from build123d import *

# Parameters (mm, degrees)
F2_R     = 5
F4_DEPTH = 1


with BuildPart() as f1:
    # F0 (on Front) → F1 (revolve)
    with BuildSketch(Plane.XZ):
        with BuildLine():
            Line((-25, 14.134617), (-25, 0))
            Line((-25, 0), (0, 0))
            Line((0, 0), (0, 35))
            ThreePointArc((0, 35), (-5.59017, 33.68034), (-10, 30))
            Line((-10, 30), (-17.5, 30))
            Line((-17.5, 30), (-17.5, 14.134617))
            Line((-17.5, 14.134617), (-25, 14.134617))
        make_face()
    revolve(axis=Axis((0, 0, 17.5), (0, 0, 1)))

    # F2
    f2_edges = [f1.edges().sort_by_distance(p)[0] for p in [
        (17.5, 0, 30),
        (25, 0, 14.134617),
    ]]
    fillet(f2_edges, radius=F2_R)

    # F3 (on face) → F4 (join)
    with BuildSketch(Plane(origin=(0, 0, 0), x_dir=(1, 0, 0), z_dir=(0, 0, -1))):
        with BuildLine():
            ThreePointArc((27.5, 0), (30, 2.5), (32.5, 0))
            Line((32.5, 0), (35, 0))
            ThreePointArc((35, 0), (34.609772, 1.936492), (33.5, 3.570714))
            Line((33.5, 3.570714), (18.2, 18.567714))
            ThreePointArc((18.2, 18.567714), (0, 26), (-18.2, 18.567714))
            Line((-18.2, 18.567714), (-33.5, 3.570714))
            ThreePointArc((-33.5, 3.570714), (-34.609772, 1.936492), (-35, 0))
            Line((-35, 0), (-32.5, 0))
            ThreePointArc((-32.5, 0), (-30, 2.5), (-27.5, 0))
            Line((-27.5, 0), (27.5, 0))
        make_face()
        with BuildLine():
            Line((35, 0), (32.5, 0))
            ThreePointArc((32.5, 0), (30, -2.5), (27.5, 0))
            Line((27.5, 0), (-27.5, 0))
            ThreePointArc((-27.5, 0), (-30, -2.5), (-32.5, 0))
            Line((-32.5, 0), (-35, 0))
            ThreePointArc((-35, 0), (-34.609772, -1.936492), (-33.5, -3.570714))
            Line((-33.5, -3.570714), (-18.2, -18.567714))
            ThreePointArc((-18.2, -18.567714), (0, -26), (18.2, -18.567714))
            Line((18.2, -18.567714), (33.5, -3.570714))
            ThreePointArc((33.5, -3.570714), (34.609772, -1.936492), (35, 0))
        make_face()
    extrude(amount=F4_DEPTH)


solid = f1.part
Read the model definition and answer for the solid it produces. Units are mm, in the model's axes. A direction names the side the tool comes from. Give positions to 0.01 mm unless a question says otherwise; leave off trailing zeros. Write each loop counter-clockwise with the first axis right and the second up, starting at its lowest first coordinate (ties: lowest second). Pieces come first, ordered by that corner, then holes. Notation, with made-up numbers: (6.25, 1.5) - (54.25, 1.5) arc R24 ccw to (54.25, 14.5) - close; hole circle Ø7 at (15, 25.5). An arc over 180 degrees is marked (long way). Return JSON: item names as keys, results as strings.
Q1. A cutting plane is placed at C-C, the plane z = 6.5. Determine the outline of the cut face in (x, y).
Reply:
{"outline": "circle Ø50 at (0, 0)"}
Q2. For faces 1 (the face through (13.887, 10.648, 19.491)), 2 (the face through (25.743, 11.174, -0.493)), determine the directions among +Z, -Z, +X, -X, +Y, -Y from which every point of the face is accessible in a straight line to the end or side of a thin tool.
Reply:
{"face 1": "+Z", "face 2": "+Z, -Z, +X, +Y"}
Q3. A cutting plane is placed at A-A, the plane x = 30. Determine the outline of the cut face in (y, z).
Reply:
{"outline": "(-7, -1) - (-2.5, -1) - (-2.5, 0) - (-7, 0) - close; (2.5, -1) - (7, -1) - (7, 0) - (2.5, 0) - close"}
Q4. Given P1, Ø12, axis at x = 17.5, z = 28, coming from the +Y side; P2, Ø12.5, axis at x = 2.5, y = 6, coming from the +Z side; P3, Ø2, axis at y = -14, z = 7, coming from the -X side; P4, Ø10, axis at x = -26.5, z = 27.5, coming from the -Y side, each flat-ended and moving along its own axis, determine where each tip first touches the part or whether it passes through.
Reply:
{"P1": "y = 12.75", "P2": "z = 35", "P3": "x = -21.35", "P4": "through"}
Q5. For a pull along Y with two mould halves and no side action, classify faces 3 (the face through (-0.3, 26, -0.5)), 4 (the face through (0, 18, 14.135)), 5 (the face through (-32.5, 0.1, -0.5)) as released by +Y, released by -Y, zero draft, split by the parting line, or undercut.
Reply:
{"face 3": "released by +Y", "face 4": "zero draft", "face 5": "undercut"}
Q6. Consider line 1 along Z through (x, y) = (5, 17); line 2 along Y through (x, z) = (-30, -0.5); line 3 along Z through (x, y) = (-22, 5.5). Determine where each line is inside the solid, lowest interval first. Write a range as [from, to].
Reply:
{"line 1": "[-1, 14.13]", "line 2": "[-7, -2.5], [2.5, 7]", "line 3": "[-1, 13.36]"}
Q7. A cutting plane is placed at B-B, the plane z = 19.5. Determine the outline of the cut face in (x, y).
Reply:
{"outline": "circle Ø35 at (0, 0)"}
